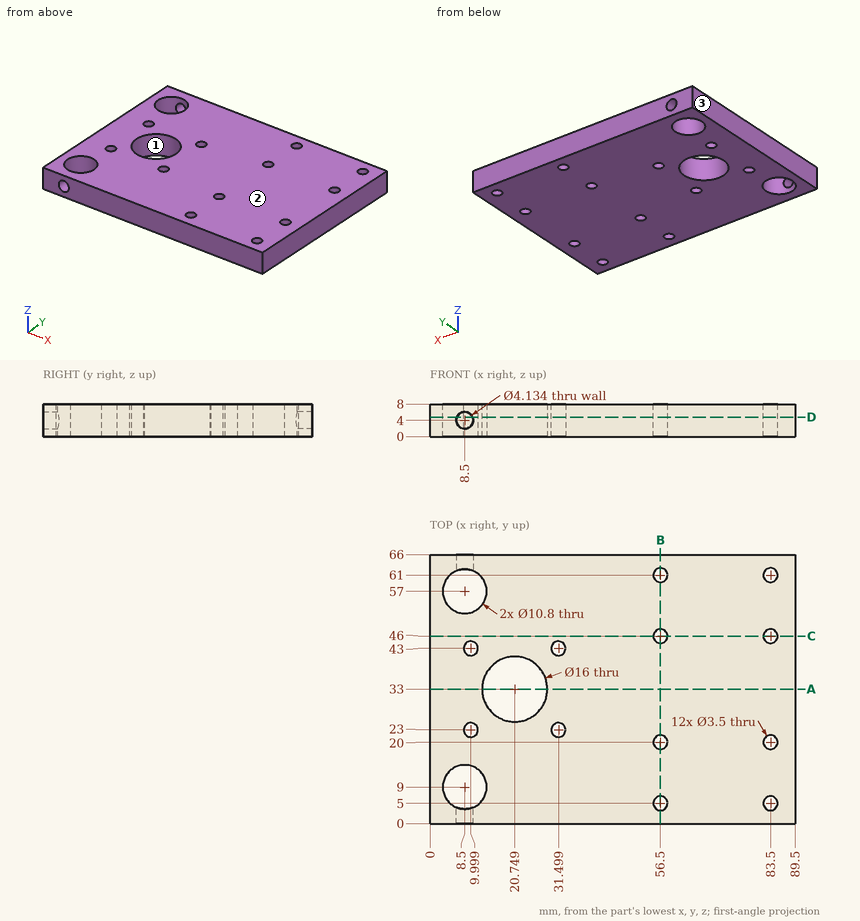
The figure shows three views and two pictorial views of one solid part (mm, origin at its lowest corner). Answer the questions. Give positions to 0.01 mm unless a question says otherwise; leave off trailing zeros. Order: outer loops, then holes, each group sorted by start corner. A loop starts at its lowest first (then second) coordinate and runs counter-clockwise, first axis right, second up. Notation, with made-up numbers: (-9.75, -33.5) -> (5.25, -33.5) arc R22 cw to (5.25, 1.5) -> close; hole circle Ø6 at (34, -5). An arc over 180 degrees is marked (long way). One line per item, written item: value.
1) Find section B-B, the plane x = 56.5. Determine the outline of the cut face in (y, z).
Reported:
outline: (0, 0) -> (3.25, 0) -> (3.25, 8) -> (0, 8) -> close; (6.75, 0) -> (18.25, 0) -> (18.25, 8) -> (6.75, 8) -> close; (21.75, 0) -> (44.25, 0) -> (44.25, 8) -> (21.75, 8) -> close; (47.75, 0) -> (59.25, 0) -> (59.25, 8) -> (47.75, 8) -> close; (62.75, 0) -> (66, 0) -> (66, 8) -> (62.75, 8) -> close
2) Determine the mould class of the marked faces 1, 2 and 3 for opening direction X: pulls with the +X half, pulls with the -X half, needs draft (parallel to the pull), parting line crosses it, or undercut.
Reported:
face 1: undercut
face 2: needs draft
face 3: pulls with the -X half
3) Find section D-D, the plane z = 4.75. Count the separate pieces of the cut face and the enclosed holes in it, plus the area to 3 significant figures.
Reported:
separate pieces: 1
enclosed holes: 13
area: 5,380 mm^2
4) Find section C-C, the plane y = 46. Determine the outline of the cut face in (x, z), plus the area to 3 significant figures.
Reported:
outline: (0, 0) -> (54.75, 0) -> (54.75, 8) -> (0, 8) -> close; (58.25, 0) -> (81.75, 0) -> (81.75, 8) -> (58.25, 8) -> close; (85.25, 0) -> (89.5, 0) -> (89.5, 8) -> (85.25, 8) -> close
area: 660 mm^2
5) Find the intervals of material crossed by line 1 (Y direction, x = 83.5, z = 5); line 2 (X direction, y = 46, z = 5.75); line 3 (X direction, y = 4.5, z = 1.75) (1 decimal), in increasing order.
Reported:
line 1: y = 0 to 3.25, 6.75 to 18.25, 21.75 to 44.25, 47.75 to 59.25, 62.75 to 66
line 2: x = 0 to 54.75, 58.25 to 81.75, 85.25 to 89.5
line 3: x = 0 to 5.5, 11.5 to 54.8, 58.2 to 81.8, 85.2 to 89.5
6) Flat-ended cylindrical pins translate along their axes: P1, Ø3, axis at x = 56.5, y = 5, coming from the +Z side; P2, Ø2.5, axis at x = 8.5, z = 4, coming from the -Y side. Find the tip coordinate at first contact, or state that the pin passes through.
Reported:
P1: passes through
P2: stops at y = 14.25
7) Find section A-A, the plane y = 33. Determine the outline of the cut face in (x, z).
Reported:
outline: (0, 0) -> (12.75, 0) -> (12.75, 8) -> (0, 8) -> close; (28.75, 0) -> (89.5, 0) -> (89.5, 8) -> (28.75, 8) -> close
